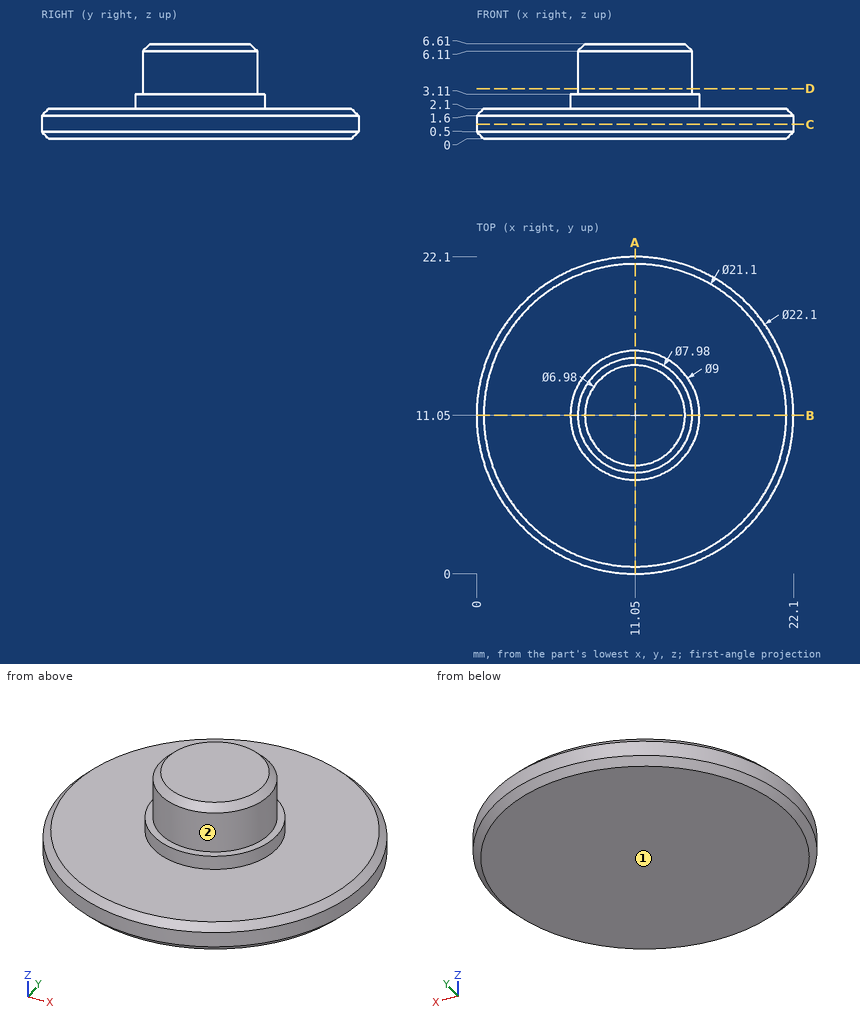
The figure shows three views and two pictorial views of one solid part (mm, origin at its lowest corner). Answer the questions. A direction names the side the tool comes from. Round coordinates to 2 decimals unless told otherwise and drop trailing zeros. Loops run counter-clockwise (first coordinate to the right, second up) from the corner with the lowest first, then second, coordinate; pieces in that order, holes last. Notation, with made-up numbers: M 88.25,-6.75 L 141.25,-6.75 A20 cw 141.25,22.25 Z; hole C 37.25,59 d3. An arc over 180 degrees is marked long. Write each question's results on one line, items separated by ' | '. Start each with the question number.
1) Find section D-D on z = 3.5. Write down the section's boundary in (x, y).
2) Straight lines are drawn through the part: probe 1 along Z at (x, y) = (5.75, 15); probe 2 along Z at (x, y) = (13.25, 14.5); probe 3 along X at (y, z) = (17, 2). For each, find the intervals that lie inside material, in ascending order.
3) Which of the six approach directions +Z, -Z, +X, -X, +Y, -Y give full straight-line access (tool end or side, diameter ignored) to the marked faces 1 and 2?
4) Find section A-A on x = 11.05. Write down the section's boundary in (y, z), plus the area to 3 significant figures.
5) Each of these flat-tipped pins is pushed along its axis until it touches: pin 1 (2 mm diameter, centred on x = 11, z = 3, fed in from +Y); pin 2 (12 mm diameter, centred on x = 20, y = 2.5, fed in from +Z). Where does it stop, or does it pass through?
6) Find section C-C on z = 1. Write down the section's boundary in (x, y).
Final values:
1) outline: C 11.05,11.05 d7.98
2) probe 1: 0 to 2.1 | probe 2: 0 to 3.11 | probe 3: 2.22 to 19.88
3) face 1: -Z, +X, -X, +Y, -Y | face 2: +Z
4) outline: M 0,0.5 L 0.5,0 L 21.6,0 L 22.1,0.5 L 22.1,1.6 L 21.6,2.1 L 15.55,2.1 L 15.55,3.11 L 15.04,3.11 L 15.04,6.11 L 14.54,6.61 L 7.56,6.61 L 7.06,6.11 L 7.06,3.11 L 6.55,3.11 L 6.55,2.1 L 0.5,2.1 L 0,1.6 Z | area: 82.7 mm²
5) pin 1: y = 21.7 | pin 2: z = 2.1
6) outline: C 11.05,11.05 d22.1
